from build123d import *

# Parameters (mm, degrees)
M3_TAPPED_HOLE1_D = 2.5


with BuildPart() as part:
    # Sketch1 → Revolve1 (revolve)
    with BuildSketch(Plane(origin=(0, 0, 0), x_dir=(0, 0, -1), z_dir=(1, 0, 0)), mode=Mode.PRIVATE) as revolve1_sk:
        Polygon((3, 4.5), (3, 1), (1.5, 1), (1.5, 0), (10, 0), (10, 2.5), (4.5, 2.5), (4.5, 4.5), align=None)
    revolve(revolve1_sk.sketch.rotate(Axis((0, 12.525252525, 0), (0, -1, 0)), 180), axis=Axis((0, 12.525252525, 0), (0, -1, 0)))

    # M3 Tapped Hole1 (through all)
    with Locations(Plane(origin=(0, 2.5, 0), x_dir=(1, 0, 0), z_dir=(0, 1, 0))):
        with Locations((0, 7), (7, 0), (0, -7), (-7, 0)):
            Hole(M3_TAPPED_HOLE1_D / 2)


solid = part.part
Input: part model. Units: mm. Frame: model coordinates. A direction names the side the tool comes from. Round coordinates to 2 decimals unless told otherwise and drop trailing zeros. Order: outer loops, then holes, each group sorted by start corner. A loop starts at its lowest first (then second) coordinate and runs counter-clockwise, first axis right, second up. Notation, with made-up numbers: (30, -16.75) - (82, -16.75) arc R27 cw to (82, 4.25) - close; hole circle Ø2 at (56.5, -3). An arc over 180 degrees is marked (long way). Answer as a JSON object with one key per item and string values. Group by question number.
(1) Material intervals for probe 1 along X at (y, z) = (0.9, -0.25); probe 2 along Y at (x, z) = (-3.5, 8.75); probe 3 along X at (y, z) = (0.9, -7), sorted ascending. Write a range as from..to.
(2) Cut plane D-D (z = -7). Return loops of the section in (x, y).
(3) Pin query (flat end, axial travel): P1, Ø7, axis at x = 0, z = 0, coming from the -Y side; P2, Ø3, axis at x = 0, z = -7, coming from the +Y side; P3, Ø3.5, axis at x = 0, z = 0, coming from the +Y side; P4, Ø1, axis at y = 0.5, z = -6, coming from the -X side. Return the tip coordinate at first contact, or that it passes through.
(4) Cut plane A-A (x = -6). Return loops of the section in (y, z).
(5) Cut plane C-C (z = 0). Return loops of the section in (x, y).
(6) Reachability of faces 1 (the face through (2.1, 2.5, 4.3)), 2 (the face through (3, 4.5, 1)) from +Z, -Z, +X, -X, +Y, -Y: full face, straight path, thin tool, end or side. Return the list, or none.
(7) Cut plane B-B (y = 2.2). Return loops of the section in (x, z).
(8) Draft query along X for faces 3 (the face through (-3.04, 3.51, -3.32)), 4 (the face through (-0.9, 2.73, 2.86)), 5 (the face through (2, 0, 0)), 6 (the face through (0.27, 1.23, -5.78)). Return one class per face: released by +X, released by -X, zero draft, split by the parting line, or undercut.
Here are the results:
{
 "1": {"probe 1": "x = -10..-8.22, -5.78..-1.48, 1.48..5.78, 8.22..10", "probe 2": "y = 0..2.5", "probe 3": "x = -7.14..-1.25, 1.25..7.14"},
 "2": {"outline": "(-7.14, 0) - (-1.25, 0) - (-1.25, 2.5) - (-7.14, 2.5) - close; (1.25, 0) - (7.14, 0) - (7.14, 2.5) - (1.25, 2.5) - close"},
 "3": {"P1": "stops at y = 0", "P2": "stops at y = 2.5", "P3": "stops at y = 1", "P4": "stops at x = -8.35"},
 "4": {"outline": "(0, -8) - (2.5, -8) - (2.5, -0.75) - (0, -0.75) - close; (0, 0.75) - (2.5, 0.75) - (2.5, 8) - (0, 8) - close"},
 "5": {"outline": "(-10, 0) - (-8.25, 0) - (-8.25, 2.5) - (-10, 2.5) - close; (-5.75, 0) - (-1.5, 0) - (-1.5, 1) - (-3, 1) - (-3, 4.5) - (-4.5, 4.5) - (-4.5, 2.5) - (-5.75, 2.5) - close; (1.5, 0) - (5.75, 0) - (5.75, 2.5) - (4.5, 2.5) - (4.5, 4.5) - (3, 4.5) - (3, 1) - (1.5, 1) - close; (8.25, 0) - (10, 0) - (10, 2.5) - (8.25, 2.5) - close"},
 "6": {"face 1": "+Y", "face 2": "+Z, -Z, +X, -X, +Y"},
 "7": {"outline": "circle Ø20 at (0, 0); hole circle Ø2.5 at (-7, 0); hole circle Ø6 at (0, 0); hole circle Ø2.5 at (0, -7); hole circle Ø2.5 at (0, 7); hole circle Ø2.5 at (7, 0)"},
 "8": {"face 3": "split by the parting line", "face 4": "undercut", "face 5": "zero draft", "face 6": "undercut"}
}
